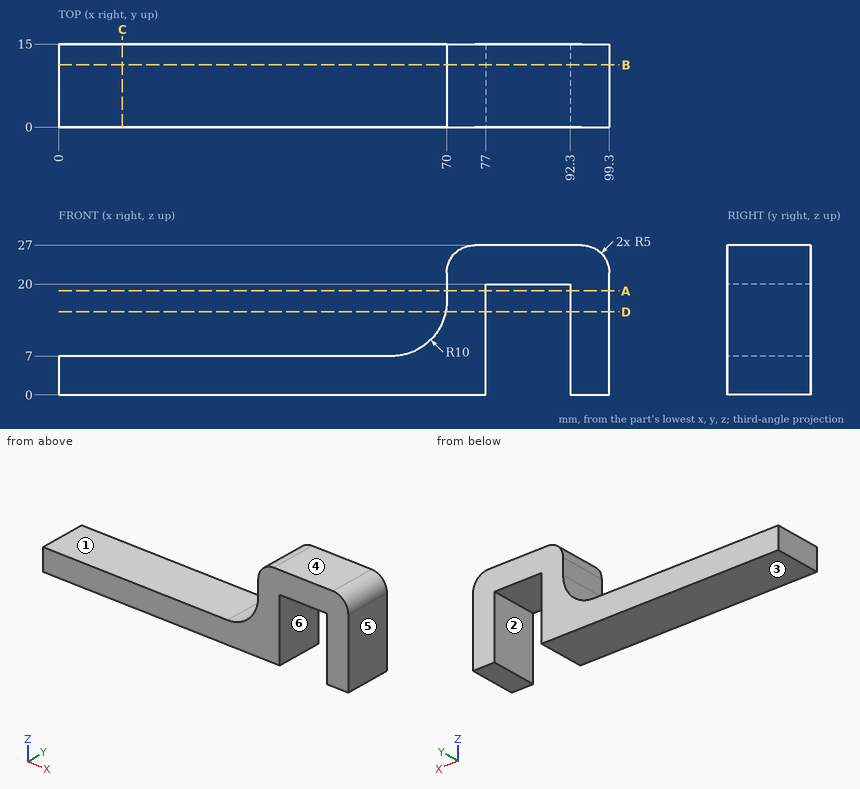
Geometry: see drawing. Coordinates: mm, zero at the bounding-box minimum. A direction names the side the tool comes from. Coordinates: 2 decimals unless noted, no trailing zeros. Order: outer loops, then holes, each group sorted by start corner. A loop starts at its lowest first (then second) coordinate and runs counter-clockwise, first axis right, second up. Notation, with made-up numbers: (-34, -19) - (-6, -19) arc R21 cw to (-6, -9) - close; hole circle Ø1 at (37, -38.5). An arc over 180 degrees is marked (long way). Use one line per item in the form item = value.
1) Section D-D (z = 15). Return loops of the section in (x, y), then the cut area to 3 significant figures.
Solutions:
outline = (69.8, 0) - (77, 0) - (77, 15) - (69.8, 15) - close; (92.3, 0) - (99.3, 0) - (99.3, 15) - (92.3, 15) - close
area = 213 mm^2
2) Section C-C (x = 11.5). Return loops of the section in (y, z), then the cut area to 3 significant figures.
Solutions:
outline = (0, 0) - (15, 0) - (15, 7) - (0, 7) - close
area = 105 mm^2
3) Set-up query: the marked faces 1, 2 and 3. Return all of +Z, -Z, +X, -X, +Y, -Y with unobstructed straight access to the full face (end or side cutting, diameter ignored); none if empty.
Solutions:
face_1 = +Z, -X, +Y, -Y
face_2 = -Z, +Y, -Y
face_3 = -Z, +X, -X, +Y, -Y
4) Section A-A (z = 18.75). Return loops of the section in (x, y).
Solutions:
outline = (70, 0) - (77, 0) - (77, 15) - (70, 15) - close; (92.3, 0) - (99.3, 0) - (99.3, 15) - (92.3, 15) - close
5) Pin query (flat end, axial travel): pin 1 (5 mm diameter, centred on x = 14, y = 9, fed in from -Z); pin 2 (4 mm diameter, centred on y = 13, z = 15.5, fed in from -X); pin 3 (1.5 mm diameter, centred on y = 4, z = 19, fed in from -X); pin 4 (1.5 mm diameter, centred on x = 87, y = 12.5, fed in from -Z). Return the tip coordinate at first contact, or that it passes through.
Solutions:
pin_1 = 0
pin_2 = 69.37
pin_3 = 70
pin_4 = 20
6) Ray query, L1, parallel to X at y = 9, z = 17.75; L2, parallel to X at y = 6.75, z = 2; L3, parallel to X at y = 6, z = 21.5. Return the intervals inside material, ascending.
Solutions:
L1 = 70 to 77, 92.3 to 99.3
L2 = 0 to 77, 92.3 to 99.3
L3 = 70 to 99.3
7) Mould query, pull axis X, two halves, no side actions, for the marked faces 4, 5 and 6. Classes: +X half, -X half, draft (parallel to the pull), parting line (faces both ways), or undercut.
Solutions:
face_4 = draft
face_5 = +X half
face_6 = undercut
8) Section B-B (y = 11.25). Return loops of the section in (x, z), then the cut area to 3 significant figures.
Solutions:
outline = (0, 0) - (77, 0) - (77, 20) - (92.3, 20) - (92.3, 0) - (99.3, 0) - (99.3, 22) arc R5 ccw to (94.3, 27) - (75, 27) arc R5 ccw to (70, 22) - (70, 17) arc R10 cw to (60, 7) - (0, 7) - close
area = 986 mm^2
